```python
from build123d import *

# Parameters (mm, degrees)
BASPROSKE_W         = 6.5
BASPROSKE_H         = 15
TOOTHCUT_DEPTH      = 23.186707732
TEETHCUTS_COUNT     = 18
TEETHCUTS_ANGLE     = 340
BORSKE_R            = 0.4
BORE_DEPTH          = 50.0000508
SKETCH_1_R          = 4.5
CUT_EXTRUDE_1_DEPTH = 2.2
SKETCH_2_R          = 1.475
CUT_EXTRUDE_2_DEPTH = 22.529170235
SKETCH_3_R          = 1.225
CUT_EXTRUDE_3_DEPTH = 23.074083695
SKETCH_4_R          = 2.15
CUT_EXTRUDE_5_DEPTH = 2.2
SKETCH_5_R          = 2.5
CUT_EXTRUDE_6_DEPTH = 3


with BuildPart() as part:
    # BasProSke → Base-Revolve (revolve)
    with BuildSketch(Plane(origin=(0, 0, 0), x_dir=(1, 0, 0), z_dir=(0, 1, 0)), mode=Mode.PRIVATE) as base_revolve_sk:
        with Locations((3.25, 7.5)):
            Rectangle(BASPROSKE_W, BASPROSKE_H)
    revolve(base_revolve_sk.sketch.rotate(Axis((-10, 0, 0), (1, 0, 0)), 180), axis=Axis((-10, 0, 0), (1, 0, 0)))

    # TooCutSke → ToothCut (cut, through all)
    with BuildSketch(Plane(origin=(0, 0, 0), x_dir=(0, 0, -1), z_dir=(1, 0, 0))):
        with BuildLine():
            ThreePointArc((0.759974923, 11.599129886), (0, 11.624), (-0.759974923, 11.599129886))
            ThreePointArc((-0.759974923, 11.599129886), (-1.229186471, 13.354767823), (-2.254227748, 14.855339189))
            ThreePointArc((-2.254227748, 14.855339189), (0, 15.0254), (2.254227748, 14.855339189))
            ThreePointArc((2.254227748, 14.855339189), (1.229186471, 13.354767823), (0.759974923, 11.599129886))
        make_face()
    toothcut = extrude(amount=TOOTHCUT_DEPTH, mode=Mode.SUBTRACT)

    # TeethCuts: ToothCut ×18 about axis
    teethcuts_axis = Axis((-10, 0, 0), (1, 0, 0))
    for i in range(1, TEETHCUTS_COUNT):
        add(toothcut.rotate(teethcuts_axis, i * TEETHCUTS_ANGLE / (TEETHCUTS_COUNT - 1)), mode=Mode.SUBTRACT)

    # BorSke → Bore (cut, symmetric)
    with BuildSketch(Plane(origin=(0, 0, 0), x_dir=(0, 0, -1), z_dir=(1, 0, 0))):
        with Locations(Location((0, 0, 0), (0, 0, 180))):
            Circle(BORSKE_R)
    extrude(amount=BORE_DEPTH, both=True, mode=Mode.SUBTRACT)

    # 草图1 → 切除-拉伸1 (cut)
    with BuildSketch(Plane(origin=(6.5, 0, 0), x_dir=(0, 0, -1), z_dir=(1, 0, 0))):
        Circle(SKETCH_1_R)
    extrude(amount=-CUT_EXTRUDE_1_DEPTH, mode=Mode.SUBTRACT)

    # 草图2 → 切除-拉伸2 (cut, through all)
    with BuildSketch(Plane(origin=(4.3, 0, 0), x_dir=(0, 0, -1), z_dir=(1, 0, 0))):
        Circle(SKETCH_2_R)
    extrude(amount=-CUT_EXTRUDE_2_DEPTH, mode=Mode.SUBTRACT)

    # 草图3 → 切除-拉伸3 (cut, through all)
    with BuildSketch(Plane(origin=(6.5, 0, 0), x_dir=(0, 0, -1), z_dir=(1, 0, 0))):
        with Locations((0, -8)):
            Circle(SKETCH_3_R)
        with Locations((0, 8)):
            Circle(SKETCH_3_R)
    extrude(amount=-CUT_EXTRUDE_3_DEPTH, mode=Mode.SUBTRACT)

    # 草图4 → 切除-拉伸5 (cut)
    with BuildSketch(Plane.ZY):
        with Locations((0, -8)):
            Circle(SKETCH_4_R)
        with Locations((0, 8)):
            Circle(SKETCH_4_R)
    extrude(amount=-CUT_EXTRUDE_5_DEPTH, mode=Mode.SUBTRACT)

    # 草图5 → 切除-拉伸6 (cut)
    with BuildSketch(Plane.ZY):
        Circle(SKETCH_5_R)
    extrude(amount=-CUT_EXTRUDE_6_DEPTH, mode=Mode.SUBTRACT)


solid = part.part
```
The model under review builds one solid part; all positions refer to its coordinate system, in mm. A direction names the side the tool comes from. Give positions to 0.01 mm unless a question says otherwise; leave off trailing zeros. Write each loop counter-clockwise with the first axis right and the second up, starting at its lowest first coordinate (ties: lowest second). Pieces come first, ordered by that corner, then holes.
(1) For P1, Ø2.5, axis at y = -1, z = 1.5, coming from the +X side; P2, Ø1, axis at x = 5, y = 2, coming from the +Z side; P3, Ø2, axis at y = -7.5, z = -0.5, coming from the -X side, all flat-tipped, find the tip position at first contact; note any pin that passes through.
(2) Consider section B-B, the plane z = 0. Give the number of separate pieces and of enclosed holes in the cut face, and give its area (3 significant figures).
(3) Consider section C-C, the plane z = -12.75. Give the boundary of the cut face in (x, y).
(4) Consider section A-A, the plane y = 0. Give the boundary of the cut face in (x, z) (3 decimals), and give its area (3 significant figures).
(5) Tool access review of faces 1 (the flat face through (4.3, -2, 0)), 2 (the cylindrical face through (3.204, -3.535, -12.946)), 3 (the cylindrical face through (3.2, 13.36, -1.23)), 4 (the flat face through (2.2, 7, 1)), 5 (the cylindrical face through (3.204, 12.929, -3.416)): name each direction out of +Z, -Z, +X, -X, +Y, -Y from which nothing blocks a thin tool from reaching the whole face with its end or side.
(6) To check wall thickness, follow L1, parallel to Y at x = 1.7, z = 0; L2, parallel to Y at x = 5.5, z = 0 (3 decimals); L3, parallel to Y at x = 3.75, z = 7. State the ranges of each line that lie inside material, in increasing order.
(7) The part is to be moulded in two halves that separate along Y. For faces 6 (the cylindrical face through (3.204, 13.318, 1.212)), 7 (the cylindrical face through (3.204, -8.911, -7.464)), 8 (the cylindrical face through (3.2, -9.44, 9.53)), say which applies: released by +Y, released by -Y, zero draft, split by the parting line, or undercut.
Returned:
1. P1: stops at x = 4.3
1. P2: stops at z = 11.53
1. P3: stops at x = 2.2
2. separate pieces: 4
2. enclosed holes: 0
2. area: 72.5 mm2
3. outline: (0, -5.64) - (6.5, -5.64) - (6.5, -3.41) - (0, -3.41) - close; (0, -1.23) - (6.5, -1.23) - (6.5, 1.23) - (0, 1.23) - close; (0, 3.41) - (6.5, 3.41) - (6.5, 5.64) - (0, 5.64) - close
4. outline: (0, -15) - (6.5, -15) - (6.5, -4.5) - (4.3, -4.5) - (4.3, -1.475) - (3, -1.475) - (3, -2.5) - (0, -2.5) - close; (0, 2.5) - (3, 2.5) - (3, 1.475) - (4.3, 1.475) - (4.3, 4.5) - (6.5, 4.5) - (6.5, 15) - (0, 15) - close
4. area: 156 mm2
5. face 1: +X
5. face 2: -Z, +X, -X
5. face 3: +X, -X, +Y
5. face 4: -X
5. face 5: +X, -X
6. L1: y = -11.62 to -10.15, -5.85 to -2.5, 2.5 to 5.85, 10.15 to 11.62
6. L2: y = -11.624 to -9.225, -6.775 to -4.5, 4.5 to 6.775, 9.225 to 11.624
6. L3: y = -13.09 to -9.56, -9.28 to 9.28, 9.56 to 13.09
7. face 6: released by +Y
7. face 7: undercut
7. face 8: released by -Y
